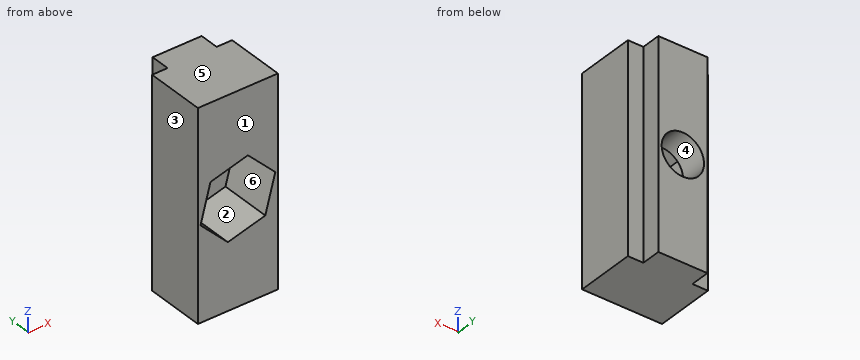
from build123d import *

# Parameters (mm, degrees)
BOSS_EXTRUDE1_DEPTH = 40
CUT_EXTRUDE1_REACH  = 17.25
SKETCH2_R           = 4.1
CUT_EXTRUDE2_DEPTH  = 10


with BuildPart() as part:
    # Sketch1 → Boss-Extrude1 (new body)
    with BuildSketch(Plane(origin=(0, 0, 0), x_dir=(0, 1, 0), z_dir=(0, 0, 1))):
        Polygon((0, 0), (0, 15.5), (11.5, 15.5), (11.5, 12.5), (15.25, 12.5), (15.25, 3), (11.5, 3), (11.5, 0), align=None)
    extrude(amount=BOSS_EXTRUDE1_DEPTH)

    # Sketch2 → Cut-Extrude1 (cut, up to next)
    with BuildSketch(Plane(origin=(0, 15.25, 0), x_dir=(-1, 0, 0), z_dir=(0, 1, 0)), mode=Mode.PRIVATE) as cut_extrude1_sk1:
        with Locations((7.75, 20)):
            Circle(SKETCH2_R)
    cut_extrude1_tool1 = extrude(cut_extrude1_sk1.sketch, amount=-CUT_EXTRUDE1_REACH, mode=Mode.PRIVATE) & part.part
    add(cut_extrude1_tool1.solids().sort_by_distance((-7.75, 15.25, 20))[0], mode=Mode.SUBTRACT)

    # Sketch3 → Cut-Extrude2 (cut)
    with BuildSketch(Plane(origin=(0, 0, 0), x_dir=(-1, 0, 0), z_dir=(0, -1, 0))):
        Polygon((2.440808402, -14.694736773), (0.500911472, -21.945263183), (5.81010307, -27.250526411), (13.059191598, -25.305263227), (14.999088528, -18.054736817), (9.68989693, -12.749473589), align=None)
    extrude(amount=-CUT_EXTRUDE2_DEPTH, mode=Mode.SUBTRACT)


solid = part.part
Verification items for the finished model (mm, model axes). Face numbers are marked on the shaded views. A direction names the side the tool comes from. Coordinates: 2 decimals unless noted, no trailing zeros. Order: outer loops, then holes, each group sorted by start corner. A loop starts at its lowest first (then second) coordinate and runs counter-clockwise, first axis right, second up. Notation, with made-up numbers: (-19, -23) -> (28, -23) arc R29 ccw to (28, 10) -> close; hole circle Ø11 at (-36.75, 4.5). An arc over 180 degrees is marked (long way). Put each result on its own line as item: value. Start each with the question number.
1. Access from +Z, -Z, +X, -X, +Y, -Y to the whole of each face (thin tool, end or side, straight path). Record for the marked faces 1 and 2.
2. Cross-section at D-D, the plane x = -11.25. Record the boundary of the cut face in (y, z).
3. Material ranges on L1, parallel to Z at x = -7.75, y = 12.9; L2, parallel to Y at x = -13, z = 24; L3, parallel to Z at x = -7, y = 5.75, recorded low to high. Write a range as [from, to].
4. Cross-section at A-A, the plane y = 2. Record the boundary of the cut face in (x, z), then the cut area to 3 significant figures.
5. Cross-section at B-B, the plane z = 20. Record the boundary of the cut face in (x, y).
6. Mould release check, pull along X, two halves, no side actions. Record for the marked faces 3, 4, 5 and 6: released by +X, released by -X, zero draft, split by the parting line, or undercut.
7. Cross-section at C-C, the plane x = -7.75. Record the boundary of the cut face in (y, z).
8. Go/stop test with flat-tipped pins: pin 1 Ø1.1 at (y, z) = (12.5, 13.5) entering from +X; pin 2 Ø1.5 at (x, z) = (-14.5, 13) entering from +Y. Record where each tip stops, or that it passes through.
Computed:
1. face 1: +Z, -Z, +X, -X, -Y
1. face 2: -Y
2. outline: (0, 0) -> (15.25, 0) -> (15.25, 17.86) -> (10, 17.86) -> (10, 14.31) -> (0, 14.31) -> close; (0, 25.79) -> (10, 25.79) -> (10, 22.14) -> (15.25, 22.14) -> (15.25, 40) -> (0, 40) -> close
3. L1: [0, 15.9], [24.1, 40]
3. L2: [10, 11.5]
3. L3: [0, 13.47], [26.93, 40]
4. outline: (-15.5, 0) -> (0, 0) -> (0, 40) -> (-15.5, 40) -> close; hole (-15, 18.05) -> (-9.69, 12.75) -> (-2.44, 14.69) -> (-0.5, 21.95) -> (-5.81, 27.25) -> (-13.06, 25.31) -> close
4. area: 474 mm2
5. outline: (-15.5, 0) -> (-14.48, 0) -> (-14.48, 10) -> (-11.85, 10) -> (-11.85, 15.25) -> (-12.5, 15.25) -> (-12.5, 11.5) -> (-15.5, 11.5) -> close; (-3.65, 10) -> (-1.02, 10) -> (-1.02, 0) -> (0, 0) -> (0, 11.5) -> (-3, 11.5) -> (-3, 15.25) -> (-3.65, 15.25) -> close
6. face 3: released by -X
6. face 4: undercut
6. face 5: zero draft
6. face 6: undercut
7. outline: (0, 0) -> (15.25, 0) -> (15.25, 15.9) -> (10, 15.9) -> (10, 13.27) -> (0, 13.27) -> close; (0, 26.73) -> (10, 26.73) -> (10, 24.1) -> (15.25, 24.1) -> (15.25, 40) -> (0, 40) -> close
8. pin 1: x = -3
8. pin 2: y = 11.5
